from build123d import *

# Parameters (mm, degrees)
F0_W     = 255
F0_H     = 100
F1_DEPTH = 60
F2_W     = 120
F2_H     = 25
F3_DEPTH = 50
F4_R     = 15
F6_D     = 2.4
F6_DEPTH = 5
F6_TIP   = 0.7210327428
F7_D     = 5
F7_DEPTH = 10
F7_TIP   = 1.5021515476


with BuildPart() as f1:
    # F0 (on Top) → F1 (new body)
    with BuildSketch(Plane.XY):
        Rectangle(F0_W, F0_H)
    extrude(amount=F1_DEPTH)

    # F2 (on face) → F3 (cut)
    with BuildSketch(Plane.XY.offset(60)):
        with Locations((-52.5, -15)):
            Rectangle(F2_W, F2_H)
    extrude(amount=-F3_DEPTH, mode=Mode.SUBTRACT)

    # F4
    f4_edges = [f1.edges().sort_by_distance(p)[0] for p in [
        (7.5, -15, 10),
        (-112.5, -15, 10),
    ]]
    fillet(f4_edges, radius=F4_R)

    # F6
    with Locations(Plane.XY.offset(60)):
        with Locations((92.5, 10), (92.5, 40), (62.5, 10), (62.5, 40), (25, 12.5), (0, 12.5), (0, 37.5), (25, 37.5), (-38.5, -32.5), (-66.5, -32.5)):
            Hole(F6_D / 2, depth=F6_DEPTH)
            with Locations((0, 0, -(F6_DEPTH + F6_TIP / 2))):  # 118° drill point
                Cone(0, F6_D / 2, F6_TIP, mode=Mode.SUBTRACT)

    # F7
    with Locations(Plane.XY.offset(60)):
        with Locations((102.5, 25)):
            Hole(F7_D / 2, depth=F7_DEPTH)
            with Locations((0, 0, -(F7_DEPTH + F7_TIP / 2))):  # 118° drill point
                Cone(0, F7_D / 2, F7_TIP, mode=Mode.SUBTRACT)


solid = f1.part
Design review of the part built by this model. Coordinates are the model's own, in mm. A direction names the side the tool comes from. Coordinates: 2 decimals unless noted, no trailing zeros. Order: outer loops, then holes, each group sorted by start corner. A loop starts at its lowest first (then second) coordinate and runs counter-clockwise, first axis right, second up. Notation, with made-up numbers: (66.5, -17.75) -> (104.5, -17.75) arc R15 ccw to (104.5, -10.75) -> close; hole circle Ø7 at (-31.75, 69.25). An arc over 180 degrees is marked (long way). Use one line per item in the form item = value. Start each with the question number.
(1) Add section A-A on z = 15.5. State the section outline as (x, y) points.
(2) The part is to be moulded in two halves that separate along Y. For faces 1 (the cylindrical face through (-108.22, -14.82, 14.51)), 2 (the flat face through (-2, 1, 60)), 3 (the flat face through (-2, 50, 30)), say which applies: +Y half, -Y half, draft (parallel to the pull), parting line (faces both ways), or undercut.
(3) For faces 4 (the flat face through (-53, -15, 10)), 5 (the flat face through (-2, 1, 0)), list the 3-axis set-ups (+Z, -Z, +X, -X, +Y, -Y) from which the entire face can be reached by the end or side of a thin tool; tool diameter is ignored.
(4) Add section B-B on y = -5. State the section outline as (x, z) points, plus the area to 3 significant figures.
(5) Add section C-C on x = -57. State the section outline as (y, z) points, plus the area to 3 significant figures.
(6) For probe 1 along Y at (x, z) = (-38.5, 56.1); probe 2 along X at (y, z) = (10, 56.8); probe 3 along Y at (x, z) = (62.5, 58.05), list the stretches that pass through material, from the lowest coordinate up.
(7) Insertion check: pin 1 (1.4 mm diameter, centred on x = 62.5, y = 10, fed in from +Z). The pin has a flat end and moves straight along its axis. Give the tip position at first contact, or say it passes through.
Answer block:
q1.outline = (-127.5, -50) -> (127.5, -50) -> (127.5, 50) -> (-127.5, 50) -> close; hole (-109.11, -27.5) -> (4.11, -27.5) -> (4.11, -2.5) -> (-109.11, -2.5) -> close
q2.face_1 = undercut
q2.face_2 = draft
q2.face_3 = +Y half
q3.face_4 = +Z
q3.face_5 = -Z, +X, -X, +Y, -Y
q4.outline = (-127.5, 0) -> (127.5, 0) -> (127.5, 60) -> (7.5, 60) -> (7.5, 25) arc R15 cw to (-7.5, 10) -> (-97.5, 10) arc R15 cw to (-112.5, 25) -> (-112.5, 60) -> (-127.5, 60) -> close
q4.area = 9,400 mm²
q5.outline = (-50, 0) -> (50, 0) -> (50, 60) -> (-2.5, 60) -> (-2.5, 10) -> (-27.5, 10) -> (-27.5, 60) -> (-50, 60) -> close
q5.area = 4,750 mm²
q6.probe_1 = -50 to -33.7, -31.3 to -27.5, -2.5 to 50
q6.probe_2 = -127.5 to 61.3, 63.7 to 91.3, 93.7 to 127.5
q6.probe_3 = -50 to 8.8, 11.2 to 38.8, 41.2 to 50
q7.pin_1 = 54.7
